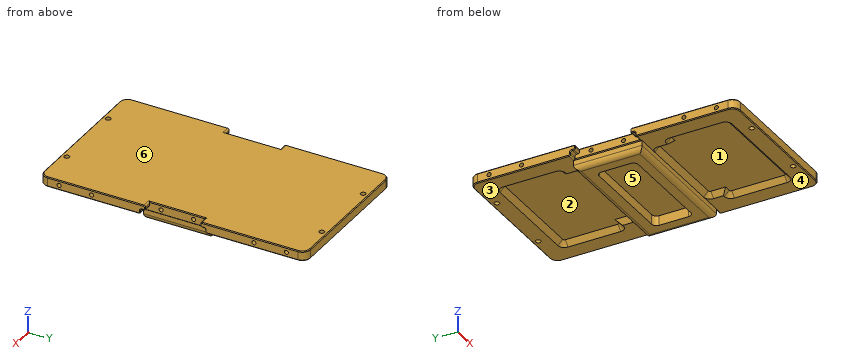
```python
from build123d import *

# Parameters (mm, degrees)
SKETCH_1_W                  = 92
SKETCH_1_H                  = 164
EXTRUDE_1_DEPTH             = 3
SKETCH_97_W                 = 3
SKETCH_97_H                 = 34
CUT_EXTRUDE_1_DEPTH         = 5
HOLE_WIZARD_M3_1_AT_2_COUNT = 2
HOLE_WIZARD_M3_1_AT_2_PITCH = 20
HOLE_WIZARD_M3_2_AT_2_COUNT = 2
HOLE_WIZARD_M3_2_AT_2_PITCH = 140
HOLE_WIZARD_M3_2_AT_3_COUNT = 2
HOLE_WIZARD_M3_2_AT_3_PITCH = 20
HOLE_WIZARD_M3_2_AT_4_COUNT = 2
HOLE_WIZARD_M3_2_AT_4_PITCH = 120
FILLET_3_R                  = 5
FILLET_5_R                  = 1
CHAMFER_2_SIZE              = 0.5
SKETCH_119_R                = 1.6
CUT_EXTRUDE_6_DEPTH         = 95.212525707
CUT_EXTRUDE_7_DEPTH         = 3
CHAMFER_3_SIZE              = 3
SKETCH_122_W                = 81
SKETCH_122_H                = 42.1
EXTRUDE_3_DEPTH             = 6
FILLET_11_R                 = 3
SKETCH_123_W                = 63
SKETCH_123_H                = 24.1
CUT_EXTRUDE_8_DEPTH         = 6
FILLET_12_R                 = 3


with BuildPart() as part:
    # 草图1 → 凸台-拉伸1 (new, symmetric)
    with BuildSketch(Plane.XY):
        Rectangle(SKETCH_1_W, SKETCH_1_H)
    extrude(amount=EXTRUDE_1_DEPTH, both=True)

    # 草图97 → 切除-拉伸1 (cut)
    with BuildSketch(Plane.ZY.offset(46)):
        Polygon((-3, -20.05), (0, -20.05), (0, -17), (0, 17), (0, 20.05), (-3, 20.05), align=None)
        with Locations((1.5, 0)):
            Rectangle(SKETCH_97_W, SKETCH_97_H)
    cut_extrude_1 = extrude(amount=-CUT_EXTRUDE_1_DEPTH, mode=Mode.SUBTRACT)

    # 草图100 → M3 螺纹孔1 (revolve, cut)
    with BuildSketch(Plane(origin=(-41, 10, 0), x_dir=(0, 0, 1), z_dir=(0, 1, 0))):
        Polygon((0, 0), (0, 7.5), (1.25, 6.748924226), (1.25, 0), align=None)
    hole_wizard_m3_1 = revolve(axis=Axis((-47.35, 10, 0), (1, 0, 0)), mode=Mode.SUBTRACT)

    # M3 螺纹孔1 at 2: M3 螺纹孔1 ×2
    with Locations(*[(0, -i * HOLE_WIZARD_M3_1_AT_2_PITCH, 0) for i in range(1, HOLE_WIZARD_M3_1_AT_2_COUNT)]):
        add(hole_wizard_m3_1, mode=Mode.SUBTRACT)

    # 镜向1: 切除-拉伸1, M3 螺纹孔1 across plane
    add(cut_extrude_1.mirror(Plane(origin=(0, 0, 0), x_dir=(0, 0, 1), z_dir=(1, 0, 0))), mode=Mode.SUBTRACT)
    add(hole_wizard_m3_1.mirror(Plane(origin=(0, 0, 0), x_dir=(0, 0, 1), z_dir=(1, 0, 0))), mode=Mode.SUBTRACT)

    # 镜向1 copy 1 sketch → 镜向1 copy 1 (revolve, cut)
    with BuildSketch(Plane(origin=(41, -10, 0), x_dir=(0, 0, 1), z_dir=(0, 1, 0))):
        Polygon((0, 0), (0, -7.5), (1.25, -6.748924226), (1.25, 0), align=None)
    revolve(axis=Axis((47.35, -10, 0), (1, 0, 0)), mode=Mode.SUBTRACT)

    # 草图113 → M3 螺纹孔2 (revolve, cut)
    with BuildSketch(Plane(origin=(-46, -70, 0), x_dir=(0, 0, 1), z_dir=(0, 1, 0))):
        Polygon((0, 0), (0, 7.5), (1.25, 6.748924226), (1.25, 0), align=None)
    hole_wizard_m3_2 = revolve(axis=Axis((-52.35, -70, 0), (1, 0, 0)), mode=Mode.SUBTRACT)

    # M3 螺纹孔2 at 2: M3 螺纹孔2 ×2
    with Locations(*[(0, i * HOLE_WIZARD_M3_2_AT_2_PITCH, 0) for i in range(1, HOLE_WIZARD_M3_2_AT_2_COUNT)]):
        add(hole_wizard_m3_2, mode=Mode.SUBTRACT)

    # M3 螺纹孔2 at 3: M3 螺纹孔2 ×2
    with Locations(*[(0, i * HOLE_WIZARD_M3_2_AT_3_PITCH, 0) for i in range(1, HOLE_WIZARD_M3_2_AT_3_COUNT)]):
        add(hole_wizard_m3_2, mode=Mode.SUBTRACT)

    # M3 螺纹孔2 at 4: M3 螺纹孔2 ×2
    with Locations(*[(0, i * HOLE_WIZARD_M3_2_AT_4_PITCH, 0) for i in range(1, HOLE_WIZARD_M3_2_AT_4_COUNT)]):
        add(hole_wizard_m3_2, mode=Mode.SUBTRACT)

    # 镜向2: M3 螺纹孔2 across plane
    add(hole_wizard_m3_2.mirror(Plane(origin=(0, 0, 0), x_dir=(0, 0, 1), z_dir=(1, 0, 0))), mode=Mode.SUBTRACT)

    # 镜向2 copy 1 sketch → 镜向2 copy 1 (revolve, cut)
    with BuildSketch(Plane(origin=(46, 70, 0), x_dir=(0, 0, 1), z_dir=(0, 1, 0))):
        Polygon((0, 0), (0, -7.5), (1.25, -6.748924226), (1.25, 0), align=None)
    revolve(axis=Axis((52.35, 70, 0), (1, 0, 0)), mode=Mode.SUBTRACT)

    # 镜向2 copy 2 sketch → 镜向2 copy 2 (revolve, cut)
    with BuildSketch(Plane(origin=(46, -50, 0), x_dir=(0, 0, 1), z_dir=(0, 1, 0))):
        Polygon((0, 0), (0, -7.5), (1.25, -6.748924226), (1.25, 0), align=None)
    revolve(axis=Axis((52.35, -50, 0), (1, 0, 0)), mode=Mode.SUBTRACT)

    # 镜向2 copy 3 sketch → 镜向2 copy 3 (revolve, cut)
    with BuildSketch(Plane(origin=(46, 50, 0), x_dir=(0, 0, 1), z_dir=(0, 1, 0))):
        Polygon((0, 0), (0, -7.5), (1.25, -6.748924226), (1.25, 0), align=None)
    revolve(axis=Axis((52.35, 50, 0), (1, 0, 0)), mode=Mode.SUBTRACT)

    # 圆角3
    fillet_3_edges = [part.edges().sort_by_distance(p)[0] for p in [
        (46, -82, 0),
        (-46, -82, 0),
        (-46, 82, 0),
        (46, 82, 0),
    ]]
    fillet(fillet_3_edges, radius=FILLET_3_R)

    # 圆角5
    fillet_5_edges = [part.edges().sort_by_distance(p)[0] for p in [
        (-43.5, -17, 0),
        (-43.5, -20.05, 0),
        (-43.5, -20.05, -3),
        (-43.5, 20.05, -3),
        (-43.5, 20.05, 0),
        (-43.5, 17, 0),
        (-43.5, 17, 3),
        (-43.5, -17, 3),
        (43.5, -20.05, 0),
        (43.5, -17, 0),
        (43.5, -17, 3),
        (43.5, 17, 3),
        (43.5, 17, 0),
        (43.5, 20.05, 0),
        (43.5, 20.05, -3),
        (43.5, -20.05, -3),
    ]]
    fillet(fillet_5_edges, radius=FILLET_5_R)

    # 倒角2
    chamfer_2_edges = [part.edges().sort_by_distance(p)[0] for p in [
        (-46, 49.025, -3),
        (-46, 47.5, 3),
        (46, -49.025, -3),
        (0, -82, -3),
        (0, 82, -3),
        (-44.535533906, -80.535533906, -3),
        (44.535533906, -80.535533906, -3),
        (44.535533906, 80.535533906, -3),
        (-44.535533906, 80.535533906, -3),
        (0, 82, 3),
        (46, -47.5, 3),
        (0, -82, 3),
        (-44.535533906, -80.535533906, 3),
        (44.535533906, -80.535533906, 3),
        (44.535533906, 80.535533906, 3),
        (-44.535533906, 80.535533906, 3),
        (-46, -20.05, -1.5),
        (-46, -49.025, -3),
        (-46, -47.5, 3),
        (-46, -17, 1.5),
        (-46, -18.525, 0),
        (-46, -17.292893219, 0.292893219),
        (-46, -17.292893219, 2.707106781),
        (-46, -20.342893219, -2.707106781),
        (46, 49.025, -3),
        (-46, 20.05, -1.5),
        (-46, 18.525, 0),
        (-46, 17, 1.5),
        (-46, 17.292893219, 0.292893219),
        (-46, 17.292893219, 2.707106781),
        (-46, 20.342893219, -2.707106781),
        (46, -20.05, -1.5),
        (46, -18.525, 0),
        (46, -17, 1.5),
        (46, -17.292893219, 0.292893219),
        (46, -17.292893219, 2.707106781),
        (46, -20.342893219, -2.707106781),
        (46, 20.05, -1.5),
        (46, 47.5, 3),
        (46, 17, 1.5),
        (46, 18.525, 0),
        (46, 17.292893219, 0.292893219),
        (46, 17.292893219, 2.707106781),
        (46, 20.342893219, -2.707106781),
        (46, -19.757106781, -0.292893219),
        (46, 19.757106781, -0.292893219),
        (-46, 19.757106781, -0.292893219),
        (-46, -19.757106781, -0.292893219),
        (-41, 0, -3),
        (-41, 0, 3),
        (41, 0, 3),
        (41, 0, -3),
    ]]
    chamfer(chamfer_2_edges, length=CHAMFER_2_SIZE)

    # 草图119 → 切除-拉伸6 (cut, through all)
    with BuildSketch(Plane(origin=(0, 0, -3), x_dir=(-1, 0, 0), z_dir=(0, 0, -1))):
        with Locations((22.5, 78.5)):
            Circle(SKETCH_119_R)
        with Locations(Location((-22.5, 78.5, 0), (0, 0, 180))):
            Circle(SKETCH_119_R)
        with Locations(Location((22.5, -78.5, 0), (0, 0, 180))):
            Circle(SKETCH_119_R)
        with Locations((-22.5, -78.5)):
            Circle(SKETCH_119_R)
    extrude(amount=-CUT_EXTRUDE_6_DEPTH, mode=Mode.SUBTRACT)

    # 草图120 → 切除-拉伸7 (cut)
    with BuildSketch(Plane(origin=(0, 0, -3), x_dir=(-1, 0, 0), z_dir=(0, 0, -1))):
        with BuildLine():
            Line((-26.5, 21.05), (26.5, 21.05))
            ThreePointArc((26.5, 21.05), (29.328427125, 22.221572875), (30.5, 25.05))
            Line((30.5, 25.05), (30.5, 31.05))
            Line((30.5, 31.05), (31.5, 31.05))
            ThreePointArc((31.5, 31.05), (34.328427125, 32.221572875), (35.5, 35.05))
            Line((35.5, 35.05), (35.5, 67.5))
            ThreePointArc((35.5, 67.5), (34.328427125, 70.328427125), (31.5, 71.5))
            Line((31.5, 71.5), (-31.5, 71.5))
            ThreePointArc((-31.5, 71.5), (-34.328427125, 70.328427125), (-35.5, 67.5))
            Line((-35.5, 67.5), (-35.5, 35.05))
            ThreePointArc((-35.5, 35.05), (-34.328427125, 32.221572875), (-31.5, 31.05))
            Line((-31.5, 31.05), (-30.5, 31.05))
            Line((-30.5, 31.05), (-30.5, 25.05))
            ThreePointArc((-30.5, 25.05), (-29.328427125, 22.221572875), (-26.5, 21.05))
        make_face()
        with BuildLine():
            Line((30.5, -31.05), (30.5, -25.05))
            ThreePointArc((30.5, -25.05), (29.328427125, -22.221572875), (26.5, -21.05))
            Line((26.5, -21.05), (-26.5, -21.05))
            ThreePointArc((-26.5, -21.05), (-29.328427125, -22.221572875), (-30.5, -25.05))
            Line((-30.5, -25.05), (-30.5, -31.05))
            Line((-30.5, -31.05), (-31.5, -31.05))
            ThreePointArc((-31.5, -31.05), (-34.328427125, -32.221572875), (-35.5, -35.05))
            Line((-35.5, -35.05), (-35.5, -67.5))
            ThreePointArc((-35.5, -67.5), (-34.328427125, -70.328427125), (-31.5, -71.5))
            Line((-31.5, -71.5), (31.5, -71.5))
            ThreePointArc((31.5, -71.5), (34.328427125, -70.328427125), (35.5, -67.5))
            Line((35.5, -67.5), (35.5, -35.05))
            ThreePointArc((35.5, -35.05), (34.328427125, -32.221572875), (31.5, -31.05))
            Line((31.5, -31.05), (30.5, -31.05))
        make_face()
    extrude(amount=-CUT_EXTRUDE_7_DEPTH, mode=Mode.SUBTRACT)

    # 倒角3
    chamfer_3_edges = [part.edges().sort_by_distance(p)[0] for p in [
        (34.328427125, 32.221572875, 0),
        (35.5, 51.275, 0),
        (34.328427125, 70.328427125, 0),
        (0, 71.5, 0),
        (-34.328427125, 70.328427125, 0),
        (-35.5, 51.275, 0),
        (-34.328427125, 32.221572875, 0),
        (-31, 31.05, 0),
        (-30.5, 28.05, 0),
        (-29.328427125, 22.221572875, 0),
        (0, 21.05, 0),
        (29.328427125, 22.221572875, 0),
        (30.5, 28.05, 0),
        (31, 31.05, 0),
        (0, -71.5, 0),
        (34.328427125, -70.328427125, 0),
        (35.5, -51.275, 0),
        (34.328427125, -32.221572875, 0),
        (31, -31.05, 0),
        (30.5, -28.05, 0),
        (29.328427125, -22.221572875, 0),
        (0, -21.05, 0),
        (-29.328427125, -22.221572875, 0),
        (-30.5, -28.05, 0),
        (-31, -31.05, 0),
        (-34.328427125, -32.221572875, 0),
        (-35.5, -51.275, 0),
        (-34.328427125, -70.328427125, 0),
    ]]
    chamfer(chamfer_3_edges, length=CHAMFER_3_SIZE - 0.0001)  # a hair under: the kernel refuses the full size

    # 草图122 → 凸台-拉伸3 (add)
    with BuildSketch(Plane(origin=(0, 0, -3), x_dir=(-1, 0, 0), z_dir=(0, 0, -1))):
        Rectangle(SKETCH_122_W, SKETCH_122_H)
    extrude(amount=EXTRUDE_3_DEPTH)

    # 圆角11
    fillet_11_edges = [part.edges().sort_by_distance(p)[0] for p in [
        (40.5, 0, -9),
        (0, -21.05, -9),
        (-40.5, 0, -9),
        (0, 21.05, -9),
    ]]
    fillet(fillet_11_edges, radius=FILLET_11_R)

    # 草图123 → 切除-拉伸8 (cut)
    with BuildSketch(Plane(origin=(0, 0, -9), x_dir=(-1, 0, 0), z_dir=(0, 0, -1))):
        Rectangle(SKETCH_123_W, SKETCH_123_H)
    extrude(amount=-CUT_EXTRUDE_8_DEPTH, mode=Mode.SUBTRACT)

    # 圆角12
    fillet_12_edges = [part.edges().sort_by_distance(p)[0] for p in [
        (-31.5, -12.05, -6),
        (31.5, -12.05, -6),
        (31.5, 12.05, -6),
        (-31.5, 12.05, -6),
    ]]
    fillet(fillet_12_edges, radius=FILLET_12_R)


solid = part.part
```
Verification items for the finished model (mm, model axes). Face numbers are marked on the shaded views. A direction names the side the tool comes from. Coordinates: 2 decimals unless noted, no trailing zeros. Write each loop counter-clockwise with the first axis right and the second up, starting at its lowest first coordinate (ties: lowest second). Pieces come first, ordered by that corner, then holes. Notation, with made-up numbers: (63, 16) - (103, 16) arc R25 cw to (103, 41) - close; hole circle Ø2 at (74.25, 28). An arc over 180 degrees is marked (long way). Write item = value, one per line.
Q1. Mould release check, pull along Y, two halves, no side actions. Record for the marked faces 1, 2 and 3: released by +Y, released by -Y, zero draft, split by the parting line, or undercut.
Answer:
face_1 = undercut
face_2 = undercut
face_3 = zero draft
Q2. Access from +Z, -Z, +X, -X, +Y, -Y to the whole of each face (thin tool, end or side, straight path). Record for the marked faces 4, 5 and 6.
Answer:
face_4 = -Z, +X, -X, -Y
face_5 = -Z
face_6 = +Z, +X, -X, +Y, -Y
Q3. Material ranges on L1, parallel to Z at x = -43.5, y = 70; L2, parallel to Z at x = -36, y = 10; L3, parallel to Y at x = 23, z = -1.75, recorded low to high. Write a range as from..to.
Answer:
L1 = -3..-1.25, 1.25..3
L2 = -9..-1.25, 1.25..3
L3 = -82..-80.02, -76.98..-70.25, -22.3..22.3, 70.25..76.98, 80.02..82
Q4. Go/stop test with flat-tipped pins: pin 1 Ø0.8 at (x, y) = (-43, -18.5) entering from -Z; pin 2 Ø1.5 at (y, z) = (-9.5, -5) entering from +X; pin 3 Ø0.9 at (x, z) = (7.5, -4.5) entering from -Y. Record where each tip stops, or that it passes through.
Answer:
pin_1 = 0
pin_2 = 40.5
pin_3 = -21.05
Q5. Cross-section at C-C (y = -2). Enter the section's corners in (x, z), plus the area to 3 significant figures.
Answer:
outline = (-41, -2.5) - (-40.5, -3) - (-40.5, -6) arc R3 ccw to (-37.5, -9) - (-31.5, -9) - (-31.5, -3) - (31.5, -3) - (31.5, -9) - (37.5, -9) arc R3 ccw to (40.5, -6) - (40.5, -3) - (41, -2.5) - (41, 2.5) - (40.5, 3) - (-40.5, 3) - (-41, 2.5) - close
area = 596 mm²
